Autodesk Inventor part; units mm, degrees
ref_plane "YZ Plane" through (0, 0, 0) normal (1, 0, 0) x (0, 1, 0)
ref_plane "XZ Plane" through (0, 0, 0) normal (0, 1, 0) x (-1, 0, 0)
ref_plane "XY Plane" through (0, 0, 0) normal (0, 0, 1) x (1, 0, 0)
sketch "Skizze1" plane through (0, 0, 0) normal (0, 0, 1) x (1, 0, 0)
  line L0 (-55.5, 96.5) -> (55.5, 96.5)
  line L1 (55.5, 96.5) -> (55.5, -96.5)
  line L2 (55.5, -96.5) -> (-55.5, -96.5)
  line L3 (-55.5, -96.5) -> (-55.5, 96.5)
  point P0 (0, 0)
  point P1 (0, 96.5)
  point P2 (-55.5, 0)
  dimension "d0" = 111
  dimension "d1" = 193
extrude "Extrusion1" add sketch "Skizze1" against normal blind 0.65
sketch "Skizze3" plane through (0, 0, 0) normal (0, 0, 1) x (1, 0, 0)
  line L0 (-42.5, 77.5) -> (44.5, 77.5)
  line L1 (44.5, 77.5) -> (44.5, -77.5)
  line L2 (44.5, -77.5) -> (-42.5, -77.5)
  line L3 (-42.5, -77.5) -> (-42.5, 77.5)
  line L4 (55.5, 96.5) -> (-55.5, 96.5)
  line L5 (-55.5, -96.5) -> (55.5, -96.5)
  line L6 (-55.5, 96.5) -> (-55.5, -96.5)
  point P0 (0, 0)
  dimension "d11" = 155
  dimension "d12" = 19
  dimension "d13" = 19
  dimension "d14" = 87
  dimension "d15" = 13
split_face "Trennen1"
fillet "Rundung1" radius 7.5 4 edges at (-55.5, -96.5, -0.325) (55.5, -96.5, -0.325) (55.5, 96.5, -0.325) (-55.5, 96.5, -0.325)
sketch "Skizze2" plane through (0, 0, -0.65) normal (0, 0, -1) x (-1, 0, 0)
  line L0 (-49, 81.5) -> (52, 81.5)
  line L1 (52, 81.5) -> (52, -85.5)
  line L2 (52, -85.5) -> (-49, -85.5)
  line L3 (-49, -85.5) -> (-49, 81.5)
  line L4 (55.5, -96.5) -> (55.5, 96.5)
  line L5 (55.5, 96.5) -> (-55.5, 96.5)
  point P0 (0, 0)
  dimension "d5" = 101
  dimension "d6" = 167
  dimension "d7" = 3.5
  dimension "d8" = 15
extrude "Extrusion2" add sketch "Skizze2" along normal blind 5.1
sketch "Skizze6" plane through (0, 0, -5.75) normal (0, 0, -1) x (-1, 0, 0)
  line L0 (-38, 68.5) -> (-30, 68.5)
  line L1 (-30, 68.5) -> (-30, 53.5)
  line L2 (-30, 53.5) -> (-38, 53.5)
  line L3 (-38, 53.5) -> (-38, 68.5)
  line L4 (28, 68.5) -> (36, 68.5)
  line L5 (36, 68.5) -> (36, 53.5)
  line L6 (36, 53.5) -> (28, 53.5)
  line L7 (28, 53.5) -> (28, 68.5)
  line L8 (-38, -57.5) -> (-30, -57.5)
  line L9 (-30, -57.5) -> (-30, -72.5)
  line L10 (-30, -72.5) -> (-38, -72.5)
  line L11 (-38, -72.5) -> (-38, -57.5)
  line L12 (28, -57.5) -> (36, -57.5)
  line L13 (36, -57.5) -> (36, -72.5)
  line L14 (36, -72.5) -> (28, -72.5)
  line L15 (28, -72.5) -> (28, -57.5)
  line L16 (-49, 81.5) -> (-49, -85.5)
  line L17 (52, 81.5) -> (-49, 81.5)
  line L18 (52, -85.5) -> (52, 81.5)
  line L19 (-49, -85.5) -> (52, -85.5)
  point P0 (0, 0)
  dimension "d35" = 8
  dimension "d36" = 15
  dimension "d37" = 11
  dimension "d38" = 13
  dimension "d39" = 16
  dimension "d40" = 13
extrude "Extrusion5" add sketch "Skizze6" along normal blind 2.5 contours L0 L1 L2 L3 | L4 L5 L6 L7 | L8 L9 L10 L11 | L12 L13 L14 L15
sketch "Skizze7" plane through (0, 0, -8.25) normal (0, 0, -1) x (-1, 0, 0)
  line L0 (-30, 68.5) -> (-38, 68.5)
  line L1 (-38, 68.5) -> (-38, 53.5)
  point P0 (0, 0)
  point P1 (-34, 61)
  point P2 (32, 61)
  point P3 (32, -65.5)
  point P4 (-34, -65.5)
  point P5 (-34, 68.5)
  point P6 (-38, 61)
  dimension "d43" = 126.5
  dimension "d44" = 66
sketch "Skizze8" plane through (38, 53.5, -5.75) normal (1, 0, 0) x (0, 0, -1)
  line L0 (0, 15) -> (2.5, 15)
  line L1 (0, 0) -> (2.5, 0)
  line L2 (0, -111) -> (2.5, -111)
  line L3 (0, -126) -> (2.5, -126)
  line L4 (2.5, -111) -> (2.5, -126)
  line L5 (0, -111) -> (2.5, -115)
  line L6 (2.5, -111) -> (2.5, -126)
  line L7 (0, -126) -> (2.5, -126)
  line L8 (0, -126) -> (2.5, -122)
  line L9 (0, 15) -> (0, 0)
  line L10 (0, 0) -> (2.5, 4)
  line L11 (2.5, 0) -> (2.5, 15)
  line L12 (0, 15) -> (2.5, 15)
  line L13 (0, 15) -> (2.5, 11)
  line L14 (0, 28) -> (0, -139)
  line L15 (0, 14.0566) -> (2, 10.8566)
  line L16 (2, 10.8566) -> (2, 4.1434)
  line L17 (2, 4.1434) -> (0, 0.9434)
  line L18 (0, -126) -> (0, -111)
  line L19 (0, -111.9434) -> (2, -115.1434)
  line L20 (2, -115.1434) -> (2, -121.8566)
  line L21 (2, -121.8566) -> (0, -125.0566)
  point P0 (-5.75, -53.5)
  point P1 (0, -111.9434)
  point P2 (0, 14.0566)
  point P3 (0, 0.9434)
  dimension "d45" = 7
  dimension "d46" = 0.5
  dimension "d47" = 0.5
  dimension "d48" = 0.5
  dimension "d49" = 0.5
extrude "Extrusion6" cut sketch "Skizze8" along normal through all both and the other way through all contours L2 L4 L5 | L0 L11 L13 | L15 L16 L17 L9 | L11 L1 L10 | L19 L20 L21 L14 | L4 L3 L8
hole "Bohrung1" at (34, 61, -8.25) at (-32, 61, -8.25) at (-32, -65.5, -8.25) at (34, -65.5, -8.25) direction (0, 0, 1) diameter 2.459 depth 0.5
sketch "Skizze4" plane through (0, 0, -5.75) normal (0, 0, -1) x (-1, 0, 0)
  line L0 (-31.5, 25) -> (24.5, 25)
  line L1 (24.5, 25) -> (24.5, -40)
  line L2 (24.5, -40) -> (-31.5, -40)
  line L3 (-31.5, -40) -> (-31.5, 25)
  line L4 (-49, -85.5) -> (52, -85.5)
  line L5 (-49, 81.5) -> (-49, -85.5)
  point P0 (0, 0)
  dimension "d17" = 45.5
  dimension "d18" = 65
  dimension "d19" = 56
  dimension "d20" = 17.5
extrude "Extrusion3" add sketch "Skizze4" along normal blind 3.45
sketch "Skizze5" plane through (0, 0, -9.2) normal (0, 0, -1) x (-1, 0, 0)
  line L0 (-26.8453, -34.5) -> (-25.6906, -36.5)
  line L1 (-25.6906, -36.5) -> (-26.8453, -38.5)
  line L2 (-26.8453, -38.5) -> (-29.1547, -38.5)
  line L3 (-29.1547, -38.5) -> (-30.3094, -36.5)
  line L4 (-30.3094, -36.5) -> (-29.1547, -34.5)
  line L5 (-29.1547, -34.5) -> (-26.8453, -34.5)
  line L6 (-26.8453, 23.5) -> (-25.6906, 21.5)
  line L7 (-25.6906, 21.5) -> (-26.8453, 19.5)
  line L8 (-26.8453, 19.5) -> (-29.1547, 19.5)
  line L9 (-29.1547, 19.5) -> (-30.3094, 21.5)
  line L10 (-30.3094, 21.5) -> (-29.1547, 23.5)
  line L11 (-29.1547, 23.5) -> (-26.8453, 23.5)
  line L12 (22.1547, 23.5) -> (23.3094, 21.5)
  line L13 (23.3094, 21.5) -> (22.1547, 19.5)
  line L14 (22.1547, 19.5) -> (19.8453, 19.5)
  line L15 (19.8453, 19.5) -> (18.6906, 21.5)
  line L16 (18.6906, 21.5) -> (19.8453, 23.5)
  line L17 (19.8453, 23.5) -> (22.1547, 23.5)
  line L18 (22.1547, -34.5) -> (23.3094, -36.5)
  line L19 (23.3094, -36.5) -> (22.1547, -38.5)
  line L20 (22.1547, -38.5) -> (19.8453, -38.5)
  line L21 (19.8453, -38.5) -> (18.6906, -36.5)
  line L22 (18.6906, -36.5) -> (19.8453, -34.5)
  line L23 (19.8453, -34.5) -> (22.1547, -34.5)
  line L24 (24.5, 25) -> (-31.5, 25)
  line L25 (-31.5, -40) -> (24.5, -40)
  line L26 (24.5, -40) -> (24.5, 25)
  line L27 (-31.5, 25) -> (-31.5, -40)
  point P0 (0, 0)
  point P1 (-28, -36.5)
  point P2 (-28, 21.5)
  point P3 (21, 21.5)
  point P4 (21, -36.5)
  point P5 (-28, 21.5)
  point P6 (21, 21.5)
  point P7 (21, -36.5)
  point P8 (-28, -36.5)
  dimension "d23" = 4
  dimension "d24" = 4
  dimension "d25" = 4
  dimension "d26" = 4
  dimension "d27" = 49
  dimension "d28" = 58
  dimension "d29" = 65
  dimension "d30" = 3.5
  dimension "d31" = 56
  dimension "d32" = 3.5
extrude "Extrusion4" add sketch "Skizze5" along normal blind 12 contours L0 L1 L2 L3 L4 L5 | L6 L7 L8 L9 L10 L11 | L12 L13 L14 L15 L16 L17 | L18 L19 L20 L21 L22 L23
equation "\"d47\" = d46"
equation "\"d48\" = d47"
equation "\"d49\" = d48"
properties part number "display"
Here's how the part is built. I have some questions about the finished solid (model axes, mm). A direction names the side the tool comes from. Coordinates: 2 decimals unless noted, no trailing zeros. Write each loop counter-clockwise with the first axis right and the second up, starting at its lowest first coordinate (ties: lowest second). Pieces come first, ordered by that corner, then holes. Notation, with made-up numbers: (-36, -34) - (-14, -34) arc R23 ccw to (-14, 4) - close; hole circle Ø1 at (64, 48). An arc over 180 degrees is marked (long way). Use one line per item in the form item = value.
1) Thinking about a two-plate mould opening in Y: for faces 4 (the flat face through (-1, 81.5, -3)), 5 (the flat face through (-33, 62, -7.75)), 6 (the flat face through (33.9, -70.5, -7)), which applies, released by +Y, released by -Y, zero draft, split by the parting line, or undercut?
Solved:
face_4 = released by +Y
face_5 = undercut
face_6 = released by -Y
2) On a 3-axis mill with a long thin cutter (end or side, diameter ignored), from which of +Z, -Z, +X, -X, +Y, -Y can I reach the whole of each face in a straight line? I mean faces 1 (the flat face through (-2, -85.5, -3)), 2 (the flat face through (-24.5, -7, -7)), 3 (the flat face through (49, -3, -3)). Say none if no direction works.
Solved:
face_1 = -Z, +X, -X, -Y
face_2 = -Z, -X, +Y, -Y
face_3 = -Z, +X, +Y, -Y
3) I need wall thicknesses on line 1 (X direction, y = 61, z = -7.95); line 2 (Y direction, x = -32, z = -8); line 3 (Y direction, x = 28, z = -19.75). Which ranges of each line are inside material? Lowest first, please.
Solved:
line_1 = -36 to -33.23, -30.77 to -28, 30 to 32.77, 35.23 to 38
line_2 = -68.9 to -66.73, -64.27 to -61.1, 57.1 to 59.77, 62.23 to 64.9
line_3 = -38.5 to -34.5, 19.5 to 23.5
4) Suppose I cut it at D-D, the plane x = 23.5. Write out the boundary of the cut face in (y, z).
Solved:
outline = (-96.5, -0.65) - (-85.5, -0.65) - (-85.5, -5.75) - (-40, -5.75) - (-40, -9.2) - (25, -9.2) - (25, -5.75) - (81.5, -5.75) - (81.5, -0.65) - (96.5, -0.65) - (96.5, 0) - (-96.5, 0) - close
5) I'm going to push flat-ended pins straight in: P1, Ø2.5, axis at y = -33, z = -4.5, coming from the -X side; P2, Ø2, axis at x = -7, y = -42.5, coming from the -Z side; P3, Ø2.5, axis at x = 28, z = -12.5, coming from the +Y side. Where does each tip first touch, or does it pass through?
Solved:
P1 = -52
P2 = -5.75
P3 = 23.5
6) Suppose I cut it at B-B, the plane y = 71.5. Write out the boundary of the cut face in (x, z).
Solved:
outline = (-55.5, -0.65) - (-52, -0.65) - (-52, -5.75) - (49, -5.75) - (49, -0.65) - (55.5, -0.65) - (55.5, 0) - (-55.5, 0) - close
7) Suppose I cut it at A-A, the plane z = -11.75. Write out the boundary of the cut face in (x, y).
Solved:
outline = (-23.31, -36.5) - (-22.15, -38.5) - (-19.85, -38.5) - (-18.69, -36.5) - (-19.85, -34.5) - (-22.15, -34.5) - close; (-23.31, 21.5) - (-22.15, 19.5) - (-19.85, 19.5) - (-18.69, 21.5) - (-19.85, 23.5) - (-22.15, 23.5) - close; (25.69, -36.5) - (26.85, -38.5) - (29.15, -38.5) - (30.31, -36.5) - (29.15, -34.5) - (26.85, -34.5) - close; (25.69, 21.5) - (26.85, 19.5) - (29.15, 19.5) - (30.31, 21.5) - (29.15, 23.5) - (26.85, 23.5) - close
8) Suppose I cut it at C-C, the plane x = 40. Write out the boundary of the cut face in (y, z), plus the area to 3 significant figures.
Solved:
outline = (-96.5, -0.65) - (-85.5, -0.65) - (-85.5, -5.75) - (81.5, -5.75) - (81.5, -0.65) - (96.5, -0.65) - (96.5, 0) - (-96.5, 0) - close
area = 977 mm2
